from build123d import *

# Parameters (mm, degrees)
BOSS_EXTRUDE1_DEPTH = 13.125
SKETCH2_R           = 7
CUT_EXTRUDE1_DEPTH  = 106.5
SKETCH2_4_R         = 11.125
SKETCH2_4_R_2       = 7
CUT_EXTRUDE2_DEPTH  = 7
SKETCH3_R           = 11.125
CUT_EXTRUDE3_DEPTH  = 7
CUT_EXTRUDE4_REACH  = 87.826
SKETCH4_R           = 7


with BuildPart() as part:
    # Sketch1 → Boss-Extrude1 (new, symmetric)
    with BuildSketch(Plane(origin=(0, 0, 0), x_dir=(1, 0, 0), z_dir=(0, 1, 0))):
        Polygon((-49.25, 13.125), (-49.25, -13.125), (-49.25, -20.400017947), (-20.400017947, -49.25), (20.400017947, -49.25), (49.25, -20.400017947), (49.25, -13.125), (49.25, 13.125), (57.25, 13.125), (57.25, -23.713726446), (23.713726446, -57.25), (-23.713726446, -57.25), (-57.25, -23.713726446), (-57.25, 13.125), align=None)
    extrude(amount=BOSS_EXTRUDE1_DEPTH, both=True)

    # Sketch2 → Cut-Extrude1 (cut)
    with BuildSketch(Plane.ZY.offset(57.25)):
        with BuildLine():
            Line((-13.125, 13.125), (-13.125, 0))
            ThreePointArc((-13.125, 0), (-12.924585281, 2.284889562), (-12.329461667, 4.5))
            ThreePointArc((-12.329461667, 4.5), (-7.523400993, 10.7547228), (0, 13.125))
            Line((0, 13.125), (-13.125, 13.125))
        make_face()
        with BuildLine():
            ThreePointArc((-12.329461667, -4.5), (-12.924585281, -2.284889562), (-13.125, 0))
            Line((-13.125, 0), (-13.125, -13.125))
            Line((-13.125, -13.125), (0, -13.125))
            ThreePointArc((0, -13.125), (-7.523400993, -10.7547228), (-12.329461667, -4.5))
        make_face()
        Circle(SKETCH2_R)
        with BuildLine():
            ThreePointArc((-5.361902647, -4.5), (-6.577739678, -2.394439545), (-7, 0))
            Line((-7, 0), (-11.125, 0))
            ThreePointArc((-11.125, 0), (-10.88472093, -2.299668513), (-10.174262873, -4.5))
            Line((-10.174262873, -4.5), (-5.361902647, -4.5))
        make_face()
        with BuildLine():
            Line((-11.125, 0), (-7, 0))
            ThreePointArc((-7, 0), (-6.577739678, 2.394439545), (-5.361902647, 4.5))
            Line((-5.361902647, 4.5), (-10.174262873, 4.5))
            ThreePointArc((-10.174262873, 4.5), (-10.88472093, 2.299668513), (-11.125, 0))
        make_face()
        with BuildLine():
            ThreePointArc((-10.174262873, -4.5), (-10.88472093, -2.299668513), (-11.125, 0))
            Line((-11.125, 0), (-13.125, 0))
            ThreePointArc((-13.125, 0), (-12.924585281, -2.284889562), (-12.329461667, -4.5))
            Line((-12.329461667, -4.5), (-10.174262873, -4.5))
        make_face()
        with BuildLine():
            Line((-13.125, 0), (-11.125, 0))
            ThreePointArc((-11.125, 0), (-10.88472093, 2.299668513), (-10.174262873, 4.5))
            Line((-10.174262873, 4.5), (-12.329461667, 4.5))
            ThreePointArc((-12.329461667, 4.5), (-12.924585281, 2.284889562), (-13.125, 0))
        make_face()
    cut_extrude1 = extrude(amount=-CUT_EXTRUDE1_DEPTH, mode=Mode.SUBTRACT)

    # Sketch2_4 → Cut-Extrude2 (cut)
    with BuildSketch(Plane.ZY.offset(57.25)):
        Circle(SKETCH2_4_R)
        Circle(SKETCH2_4_R_2, mode=Mode.SUBTRACT)
    cut_extrude2 = extrude(amount=-CUT_EXTRUDE2_DEPTH, mode=Mode.SUBTRACT)

    # Mirror1: Cut-Extrude1, Cut-Extrude2 across plane
    add(cut_extrude1.mirror(Plane(origin=(0, 0, 0), x_dir=(0, 0, 1), z_dir=(1, 0, 0))), mode=Mode.SUBTRACT)
    add(cut_extrude2.mirror(Plane(origin=(0, 0, 0), x_dir=(0, 0, 1), z_dir=(1, 0, 0))), mode=Mode.SUBTRACT)

    # Sketch3 → Cut-Extrude3 (cut)
    with BuildSketch(Plane.XY.offset(57.25)):
        Circle(SKETCH3_R)
    extrude(amount=-CUT_EXTRUDE3_DEPTH, mode=Mode.SUBTRACT)

    # Sketch4 → Cut-Extrude4 (cut, up to next)
    with BuildSketch(Plane.XY.offset(50.25), mode=Mode.PRIVATE) as cut_extrude4_sk1:
        Circle(SKETCH4_R)
    cut_extrude4_tool1 = extrude(cut_extrude4_sk1.sketch, amount=-CUT_EXTRUDE4_REACH, mode=Mode.PRIVATE) & part.part
    add(cut_extrude4_tool1.solids().sort_by_distance((0, 0, 50.25))[0], mode=Mode.SUBTRACT)


solid = part.part
Build history of the part. All positions in model axes, mm. A direction names the side the tool comes from. Give positions to 0.01 mm unless a question says otherwise; leave off trailing zeros. Order: outer loops, then holes, each group sorted by start corner. A loop starts at its lowest first (then second) coordinate and runs counter-clockwise, first axis right, second up. Notation, with made-up numbers: M -14.75,53.5 L 19.25,53.5 A26 cw 19.25,76.5 Z; hole C 72,-10 d5. An arc over 180 degrees is marked long. Put each result on its own line as item: value.
Item 1: Slice it at D-D, the plane x = 16. Write the cut outline in (y, z) (3 decimals), plus the area to 3 significant figures.
From the geometry:
outline: M -13.125,49.25 L 13.125,49.25 L 13.125,57.25 L -13.125,57.25 Z
area: 210 mm2
Item 2: Slice it at A-A, the plane x = 0. Write the cut outline in (y, z) (3 decimals), plus the area to 4 significant figures.
From the geometry:
outline: M -13.125,49.25 L -7,49.25 L -7,50.25 L -11.125,50.25 L -11.125,57.25 L -13.125,57.25 Z; M 7,49.25 L 13.125,49.25 L 13.125,57.25 L 11.125,57.25 L 11.125,50.25 L 7,50.25 Z
area: 40.25 mm2
Item 3: Slice it at B-B, the plane y = -2. Write the cut outline in (x, z).
From the geometry:
outline: M -57.25,10.94 L -50.25,10.94 L -50.25,6.71 L -49.25,6.71 L -49.25,20.4 L -20.4,49.25 L -6.71,49.25 L -6.71,50.25 L -10.94,50.25 L -10.94,57.25 L -23.71,57.25 L -57.25,23.71 Z; M 6.71,49.25 L 20.4,49.25 L 49.25,20.4 L 49.25,6.71 L 50.25,6.71 L 50.25,10.94 L 57.25,10.94 L 57.25,23.71 L 23.71,57.25 L 10.94,57.25 L 10.94,50.25 L 6.71,50.25 Z
Item 4: Two-plate mould, pull along X, no slides. Class faces 5 (the flat face through (-0.2, -7.3, 50.25)), 6 (the cylindrical face through (-50, 0, 7)), 7 (the flat face through (50.25, 0.2, 7.4)): +X half, -X half, draft (parallel to the pull), parting line (faces both ways), or undercut.
From the geometry:
face 5: undercut
face 6: draft
face 7: +X half
Item 5: 3-axis set-ups, long thin cutter, end or side, ignore diameter. For faces 1 (the cylindrical face through (53.799, -0.424, 11.117)), 2 (the cylindrical face through (-53.799, -0.424, 11.117)), 3 (the flat face through (-5, 6, 49.25)), 4 (the flat face through (52.42, 4.5, -10.35)): which of +Z, -Z, +X, -X, +Y, -Y reach the whole face in a straight line?
From the geometry:
face 1: +X
face 2: -X
face 3: -Z, +Y, -Y
face 4: -Z, +X, -X
Item 6: Probe line 1 (X direction, y = 11.25, z = -6); line 2 (Y direction, x = 55, z = 0) (3 decimals); line 3 (X direction, y = 6.25, z = 22.5). List the from-to ranges inside material, lowest first. Write a range as [from, to].
From the geometry:
line 1: x = [-57.25, -49.25], [49.25, 57.25]
line 2: y = [-13.125, -11.125], [11.125, 13.125]
line 3: x = [-57.25, -47.15], [47.15, 57.25]
Item 7: Flat gauge pins, fed straight in: pin 1 Ø10 at (y, z) = (0.5, 5) entering from -X; pin 2 Ø11 at (y, z) = (0, 0) entering from +X; pin 3 Ø3.5 at (x, z) = (-54.5, -7.5) entering from -Y; pin 4 Ø7.5 at (x, z) = (51.5, -7.5) entering from +Y. Where does each tip first touch, or does it go through?
From the geometry:
pin 1: stops at x = -50.25
pin 2: passes through
pin 3: stops at y = -11.8
pin 4: stops at y = 12.58
Item 8: Slice it at C-C, the plane z = 33.5. Write the cut outline in (x, y) (3 decimals), plus the area to 3 significant figures.
From the geometry:
outline: M -47.464,-13.125 L -36.15,-13.125 L -36.15,13.125 L -47.464,13.125 Z; M 36.15,-13.125 L 47.464,-13.125 L 47.464,13.125 L 36.15,13.125 Z
area: 594 mm2
